Verification items for the finished model (mm, model axes). A direction names the side the tool comes from. Round coordinates to 2 decimals unless told otherwise and drop trailing zeros. Order: outer loops, then holes, each group sorted by start corner. A loop starts at its lowest first (then second) coordinate and runs counter-clockwise, first axis right, second up. Notation, with made-up numbers: M 78,13 L 121,13 A14 ccw 121,28 Z; hole C 3,16.5 d2. An arc over 180 degrees is marked long. Use CSV: the item, a comma, the result in double quotes. Start each with the question number.
Q1. Set-up check for faces 1 (the face through (-6, 1, -3.81)), 2 (the face through (1, 4, -3.81)), 3 (the face through (-1.27, 7, 0)), 4 (the face through (-4, 4.572, 0)), 5 (the face through (1, 4, 3.81)): record each of +Z, -Z, +X, -X, +Y, -Y from which the full face is reachable in a straight line by a thin tool's end or side.
Q2. Sectioned sample at A-A (z = -2.25). Enter the section's corners in (x, y), and give its area (3 significant figures).
Q3. Sectioned sample at B-B (x = 10.16). Enter the section's corners in (y, z).
Q4. Gauge pin test, flat ends, axial feed: pin 1 Ø2 at (x, y) = (3, 6.5) entering from +Z; pin 2 Ø1 at (x, y) = (6.5, 3.5) entering from -Z; pin 3 Ø2.5 at (x, z) = (-10.16, 0) entering from +Y; pin 4 Ø2 at (x, z) = (-4, 1.5) entering from +Y. Record the tip position at first contact, or that the pin passes through.
Q5. Mould release check, pull along X, two halves, no side actions. Record for faces 6 (the face through (7.62, 4, 0)), 7 (the face through (9.39, 1.25, 0.7)), 8 (the face through (-5.334, 2, 0)), 9 (the face through (0, 1, 6.35)): +X half, -X half, draft (parallel to the pull), parting line (faces both ways), or undercut.
Q6. Sectioned sample at C-C (z = 0). Enter the section's corners in (x, y), and give its area (3 significant figures).
Q7. Scan lines: line 1 (Z direction, x = -10.16, y = 1.35); line 2 (Y direction, x = -3.75, z = 1.75); line 3 (Y direction, x = -1, z = 4.75). Record each from-to range of solid material in increasing order.
Q8. Sectioned sample at D-D (x = -4.5). Enter the section's corners in (y, z), and give its area (3 significant figures).
```python
from build123d import *

# Parameters (mm, degrees)
SKETCH1_W           = 25.4
SKETCH1_H           = 12.7
BOSS_EXTRUDE1_DEPTH = 2.54
SKETCH2_W           = 15.24
SKETCH2_H           = 7.62
BOSS_EXTRUDE2_DEPTH = 2.032
SKETCH3_R           = 1.0414
CUT_EXTRUDE1_DEPTH  = 5.572
SKETCH4_W           = 2.286
SKETCH4_H           = 7.62
CUT_EXTRUDE2_DEPTH  = 4.572
SKETCH5_W           = 1.524
SKETCH5_H           = 7.62
BOSS_EXTRUDE3_DEPTH = 5.08


with BuildPart() as part:
    # Sketch1 → Boss-Extrude1 (new body)
    with BuildSketch(Plane(origin=(0, 0, 0), x_dir=(1, 0, 0), z_dir=(0, 1, 0))):
        Rectangle(SKETCH1_W, SKETCH1_H)
    extrude(amount=BOSS_EXTRUDE1_DEPTH)

    # Sketch2 → Boss-Extrude2 (add)
    with BuildSketch(Plane(origin=(0, 2.54, 0), x_dir=(1, 0, 0), z_dir=(0, 1, 0))):
        Rectangle(SKETCH2_W, SKETCH2_H)
    extrude(amount=BOSS_EXTRUDE2_DEPTH)

    # Sketch3 → Cut-Extrude1 (cut, through all)
    with BuildSketch(Plane.XZ):
        with Locations((-10.16, 0)):
            Circle(SKETCH3_R)
        with Locations((10.16, 0)):
            Circle(SKETCH3_R)
    extrude(amount=-CUT_EXTRUDE1_DEPTH, mode=Mode.SUBTRACT)

    # Sketch4 → Cut-Extrude2 (cut)
    with BuildSketch(Plane(origin=(0, 4.572, 0), x_dir=(1, 0, 0), z_dir=(0, 1, 0))):
        with Locations((-6.477, 0)):
            Rectangle(SKETCH4_W, SKETCH4_H)
    extrude(amount=-CUT_EXTRUDE2_DEPTH, mode=Mode.SUBTRACT)

    # Sketch5 → Boss-Extrude3 (add)
    with BuildSketch(Plane(origin=(0, 4.572, 0), x_dir=(1, 0, 0), z_dir=(0, 1, 0))):
        with Locations((-2.032, 0)):
            Rectangle(SKETCH5_W, SKETCH5_H)
    extrude(amount=BOSS_EXTRUDE3_DEPTH)


solid = part.part
```
Verdict:
1,face 1,"+Y, -Y"
1,face 2,"-Z, +X, -X, +Y"
1,face 3,"+Z, -Z, +X, +Y"
1,face 4,"+Z, -Z, -X, +Y"
1,face 5,"+Z, +X, -X, +Y"
2,outline,"M -12.7,0 L -7.62,0 L -7.62,2.54 L -12.7,2.54 Z; M -5.33,0 L 12.7,0 L 12.7,2.54 L 7.62,2.54 L 7.62,4.57 L -1.27,4.57 L -1.27,9.65 L -2.79,9.65 L -2.79,4.57 L -5.33,4.57 Z"
2,area,"92.8 mm²"
3,outline,"M 0,-6.35 L 2.54,-6.35 L 2.54,-1.04 L 0,-1.04 Z; M 0,1.04 L 2.54,1.04 L 2.54,6.35 L 0,6.35 Z"
4,pin 1,"passes through"
4,pin 2,"stops at z = -3.81"
4,pin 3,"stops at y = 2.54"
4,pin 4,"stops at y = 4.57"
5,face 6,"+X half"
5,face 7,"undercut"
5,face 8,"undercut"
5,face 9,"draft"
6,outline,"M -12.7,0 L -11.2,0 L -11.2,2.54 L -12.7,2.54 Z; M -9.12,0 L -7.62,0 L -7.62,2.54 L -9.12,2.54 Z; M -5.33,0 L 9.12,0 L 9.12,2.54 L 7.62,2.54 L 7.62,4.57 L -1.27,4.57 L -1.27,9.65 L -2.79,9.65 L -2.79,4.57 L -5.33,4.57 Z; M 11.2,0 L 12.7,0 L 12.7,2.54 L 11.2,2.54 Z"
6,area,"82.2 mm²"
7,line 1,"z = -6.35 to -1.04, 1.04 to 6.35"
7,line 2,"y = 0 to 4.57"
7,line 3,"y = 0 to 2.54"
8,outline,"M 0,-6.35 L 2.54,-6.35 L 2.54,-3.81 L 4.57,-3.81 L 4.57,3.81 L 2.54,3.81 L 2.54,6.35 L 0,6.35 Z"
8,area,"47.7 mm²"
